For this review, use the dimensioned drawing (mm, ordinates from the lowest corner) and the shaded views. Give positions to 0.01 mm unless a question says otherwise; leave off trailing zeros. Order: outer loops, then holes, each group sorted by start corner. A loop starts at its lowest first (then second) coordinate and runs counter-clockwise, first axis right, second up. Notation, with made-up numbers: M 62.25,41 L 88.25,41 A25 cw 88.25,53 Z; hole C 88,-31.5 d10. An arc over 180 degrees is marked long. Answer as CSV lines item,"result". Start each with the question number.
1. We need section A-A, the plane z = 11.25. Give the boundary of the cut face in (x, y).
2. We need section D-D, the plane x = 15. Give the boundary of the cut face in (y, z), and give its area (3 significant figures).
3. We need section B-B, the plane y = 1.9. Give the boundary of the cut face in (x, z), and give its area (3 significant figures).
4. For line 1 along X through (y, z) = (2.45, 2.5); line 2 along X through (y, z) = (2.8, 10); line 3 along Z through (x, y) = (171.5, 2.05), list the stretches that pass through material, from the lowest coordinate up.
5. Clearance check with flat-ended pins moving along their axes: P1, Ø1, axis at y = 1.5, z = 6, coming from the -X side; P2, Ø3, axis at x = 69.5, z = 3, coming from the -Y side; P3, Ø1.5, axis at y = 1, z = 2, coming from the -X side; P4, Ø1.5, axis at x = 92, y = 2, coming from the +Z side. State where each tip first meets the part, or that it passes through.
6. We need section C-C, the plane z = 1.5. Give the boundary of the cut face in (x, y), and give its area (3 significant figures).
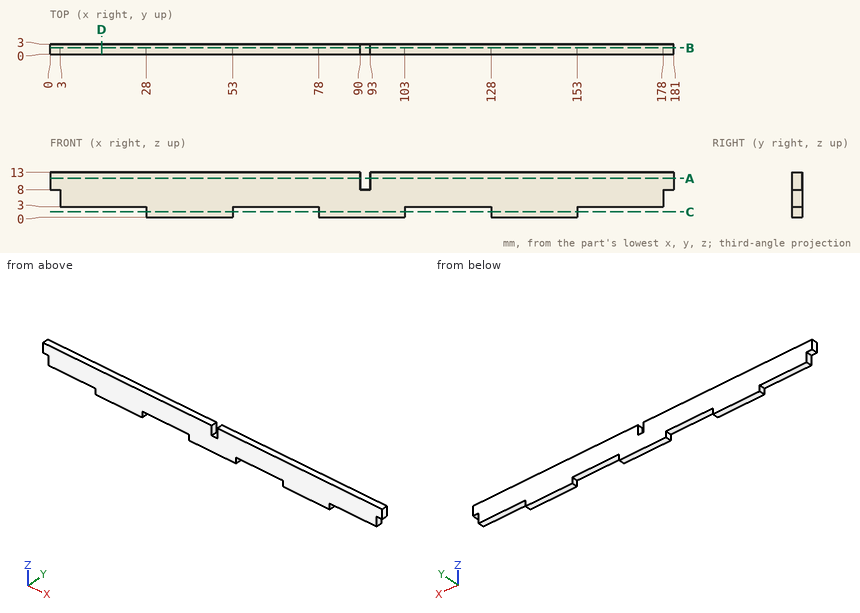
Result set:
1,outline,"M 0,0 L 90,0 L 90,3 L 0,3 Z; M 93,0 L 181,0 L 181,3 L 93,3 Z"
2,outline,"M 0,3 L 3,3 L 3,13 L 0,13 Z"
2,area,"30.0 mm2"
3,outline,"M 0,8 L 3,8 L 3,3 L 28,3 L 28,0 L 53,0 L 53,3 L 78,3 L 78,0 L 103,0 L 103,3 L 128,3 L 128,0 L 153,0 L 153,3 L 178,3 L 178,8 L 181,8 L 181,13 L 93,13 L 93,8 L 90,8 L 90,13 L 0,13 Z"
3,area,"1,990 mm2"
4,line 1,"28 to 53, 78 to 103, 128 to 153"
4,line 2,"0 to 90, 93 to 181"
4,line 3,"3 to 13"
5,P1,"x = 3"
5,P2,"y = 0"
5,P3,"x = 28"
5,P4,"z = 8"
6,outline,"M 28,0 L 53,0 L 53,3 L 28,3 Z; M 78,0 L 103,0 L 103,3 L 78,3 Z; M 128,0 L 153,0 L 153,3 L 128,3 Z"
6,area,"225 mm2"
